Can you work these out from the model? Positions are in its coordinate system, mm. A direction names the side the tool comes from. Give positions to 0.01 mm unless a question says otherwise; leave off trailing zeros. Write each loop counter-clockwise with the first axis right and the second up, starting at its lowest first coordinate (ties: lowest second). Pieces come first, ordered by that corner, then holes.
from build123d import *

# Parameters (mm, degrees)
F1_W            = 12
F1_H            = 42
F2_DEPTH        = 12
F7_R            = 11.5
F7_R_2          = 3.775
F9_DEPTH        = 25
F8_R            = 5.05
F10_DEPTH       = 0.4
F11_D           = 4.8
F12_D           = 3.5
F12_CBORE_D     = 6.2
F12_CBORE_DEPTH = 9
F14_DEPTH       = 25
F16_DEPTH       = 25
F17_SIZE        = 5
F18_T1_DEPTH    = 22.2867319519
F19_R           = 1
F20_R           = 4.5
F21_DEPTH       = 3.1
F22_R           = 10


# Not quite as in the source:
# - a fillet or chamfer that OpenCascade refuses, or shapes differently, is made with other operations: its cross-section is extruded or revolved along the edge and cut away or added


with BuildPart() as f2:
    # F1 (on Top) → F2 (new body)
    with BuildSketch(Plane.XY):
        with Locations((-6, 21)):
            Rectangle(F1_W, F1_H)
    extrude(amount=F2_DEPTH)

    # F7 (on offset) → F9 (cut)
    with BuildSketch(Plane.XY.offset(1.5)):
        with Locations((-6.5, 21)):
            Circle(F7_R)
        with Locations((-6.5, 21)):
            Circle(F7_R_2, mode=Mode.SUBTRACT)
    extrude(amount=F9_DEPTH, mode=Mode.SUBTRACT)

    # F8 (on offset) → F10 (join)
    with BuildSketch(Plane.XY.offset(1.5)):
        with Locations((-6.5, 21)):
            Circle(F8_R)
    extrude(amount=F10_DEPTH)

    # F11 (through all)
    with Locations(Plane(origin=(0, 0, 0), x_dir=(1, 0, 0), z_dir=(0, 0, -1))):
        with Locations((-6.5, -21)):
            Hole(F11_D / 2)

    # F12 (through all)
    with Locations(Plane.XY.offset(12)):
        with Locations((-6.3, 5.6)):
            CounterBoreHole(F12_D / 2, F12_CBORE_D / 2, F12_CBORE_DEPTH)

    # F13 (on Top) → F14 (cut)
    with BuildSketch(Plane.XY):
        Polygon((-5, 42), (-4, 30), (0, 19.4664706794), (0, 42), align=None)
    extrude(amount=F14_DEPTH, mode=Mode.SUBTRACT)

    # F15 (on offset) → F16 (cut)
    with BuildSketch(Plane(origin=(-12, 0, 0), x_dir=(0, -1, 0), z_dir=(-1, 0, 0))):
        with BuildLine():
            Line((-36.75, 6.6), (-38.65, 6.6))
            ThreePointArc((-38.65, 6.6), (-39.9227922061, 6.0727922061), (-40.45, 4.8))
            Line((-40.45, 4.8), (-40.45, 4.7))
            ThreePointArc((-40.45, 4.7), (-39.9227922061, 3.4272077939), (-38.65, 2.9))
            Line((-38.65, 2.9), (-36.75, 2.9))
            ThreePointArc((-36.75, 2.9), (-35.4772077939, 3.4272077939), (-34.95, 4.7))
            Line((-34.95, 4.7), (-34.95, 4.8))
            ThreePointArc((-34.95, 4.8), (-35.4772077939, 6.0727922061), (-36.75, 6.6))
        make_face()
    extrude(amount=-F16_DEPTH, mode=Mode.SUBTRACT)

    # F17
    f17_edges = [f2.edges().sort_by_distance(p)[0] for p in [
        (-12, 0, 6),
    ]]
    chamfer(f17_edges, length=F17_SIZE)

    # F18: chamfer of 2 on 1 edges, made by hand

    # F18_s2 → F18_t1 (cut)
    with BuildSketch(Plane.XY.offset(-5.1433659759)):
        Polygon((-12, 40), (-10, 42), (-12, 42), align=None)
    extrude(amount=F18_T1_DEPTH, mode=Mode.SUBTRACT)

    # F19
    f19_edges = [f2.edges().sort_by_distance(p)[0] for p in [
        (0, 0, 6),
        (-5, 42, 6),
    ]]
    fillet(f19_edges, radius=F19_R)

    # F20 (on offset) → F21 (cut)
    with BuildSketch(Plane.XY.offset(12)):
        with Locations((-6.5, 21)):
            Circle(F20_R)
    extrude(amount=-F21_DEPTH, mode=Mode.SUBTRACT)

    # F22
    f22_edges = [f2.edges().sort_by_distance(p)[0] for p in [
        (-4, 30, 0.75),
        (0, 19.466471, 0.75),
    ]]
    fillet(f22_edges, radius=F22_R)


solid = f2.part
(1) For faces 1 (the face through (-5.7, 18.5, 8.9)), 2 (the face through (-3.79, 25.26, 1.7)), 3 (the face through (-3.9, 30, 0.8)), 4 (the face through (-8, 37, 12)), 5 (the face through (-8.259, 35.463, 6.059)), which set-ups out of +Z, -Z, +X, -X, +Y, -Y let a thin tool reach every point of the face, with its end or its side?
Returned:
face 1: +Z, +X, -X
face 2: +Z
face 3: +Z, -Z, +X, +Y
face 4: +Z, +X, -X, +Y, -Y
face 5: +X, -X
(2) Will these pins go through, and if not, where does the flat tip stop? P1, Ø4.5, axis at x = -6.5, y = 21, coming from the +Z side; P2, Ø6, axis at x = -4, y = 17.5, coming from the +Z side.
Returned:
P1: passes through
P2: stops at z = 8.9
(3) Imagine slicing it at B-B, the plane z = 7.5. Give the number of separate pieces and of enclosed holes in the cut face, plus the area to 3 significant figures.
Returned:
separate pieces: 3
enclosed holes: 2
area: 175 mm2
(4) If I drill on L1, parallel to Z at x = -10.75, y = 37.5; L2, parallel to X at y = 21, z = 2.5 (3 decimals); L3, parallel to Y at x = -6.5, z = 3.25 (3 decimals), over which ranges is the centre line in solid material (lowest first)?
Returned:
L1: z = 0 to 2.9, 6.6 to 12
L2: x = -10.275 to -8.9, -4.1 to -2.725
L3: y = 0 to 2.506, 8.694 to 9.5, 17.225 to 18.6, 23.4 to 24.775, 32.5 to 35.683, 39.717 to 42
(5) If we mould it in two halves opening along X, with no side actions, what happens to faces 6 (the face through (-5.01, 6.78, 1.48)), 7 (the face through (-8, 38, 2.9)), 8 (the face through (-11, 41, 6))? For each: +X half, -X half, draft (parallel to the pull), parting line (faces both ways), or undercut.
Returned:
face 6: undercut
face 7: draft
face 8: -X half
(6) Imagine slicing it at A-A, the plane y = 5.6. Write out the boundary of the cut face in (x, z), plus the area to 3 significant figures.
Returned:
outline: (-12, 0) - (-8.05, 0) - (-8.05, 3) - (-9.4, 3) - (-9.4, 12) - (-12, 12) - close; (-4.55, 0) - (0, 0) - (0, 12) - (-3.2, 12) - (-3.2, 3) - (-4.55, 3) - close
area: 77.7 mm2
